```python
from build123d import *

# Parameters (mm, degrees)
SKETCH_1_W          = 56
SKETCH_1_H          = 85
SKETCH_1_R          = 1.5
EXTRUDE_1_DEPTH     = 1.28
FILLET_1_R          = 3
SKETCH_6_W          = 5
SKETCH_6_H          = 6
CUT_EXTRUDE_1_DEPTH = 2.28
SKETCH_4_W          = 8
SKETCH_4_H          = 10
EXTRUDE_2_DEPTH     = 6
SKETCH_5_W          = 9
SKETCH_5_H          = 4
EXTRUDE_3_DEPTH     = 3
SKETCH_2_W          = 13
SKETCH_2_H          = 13
EXTRUDE_4_DEPTH     = 7
SKETCH_3_W          = 7
SKETCH_3_H          = 8
EXTRUDE_5_DEPTH     = 3
SKETCH_7_W          = 1.5
SKETCH_7_H          = 1.5
EXTRUDE_6_DEPTH     = 2
EXTRUDE_START       = 37.5
EXTRUDE_8_DEPTH     = 67


with BuildPart() as part:
    # 草圖1 → 填料-伸長1 (new body)
    with BuildSketch(Plane(origin=(0, 0, 0), x_dir=(1, 0, 0), z_dir=(0, 1, 0))):
        Rectangle(SKETCH_1_W, SKETCH_1_H)
        with Locations((-24.5, 19)):
            Circle(SKETCH_1_R, mode=Mode.SUBTRACT)
        with Locations((-24.5, -39)):
            Circle(SKETCH_1_R, mode=Mode.SUBTRACT)
        with Locations((24.5, -39)):
            Circle(SKETCH_1_R, mode=Mode.SUBTRACT)
        with Locations((24.5, 19)):
            Circle(SKETCH_1_R, mode=Mode.SUBTRACT)
    extrude(amount=EXTRUDE_1_DEPTH)

    # 圓角1
    fillet_1_edges = [part.edges().sort_by_distance(p)[0] for p in [
        (28, 0.64, 42.5),
        (-28, 0.64, 42.5),
        (-28, 0.64, -42.5),
        (28, 0.64, -42.5),
    ]]
    fillet(fillet_1_edges, radius=FILLET_1_R)

    # 草圖6 → 除料-伸長1 (cut, through all)
    with BuildSketch(Plane(origin=(0, 1.28, 0), x_dir=(1, 0, 0), z_dir=(0, 1, 0))):
        with Locations((-23.1, -29.5)):
            Rectangle(SKETCH_6_W, SKETCH_6_H)
    extrude(amount=-CUT_EXTRUDE_1_DEPTH, mode=Mode.SUBTRACT)

    # 草圖4 → 填料-伸長2 (add)
    with BuildSketch(Plane(origin=(0, 1.28, 0), x_dir=(1, 0, 0), z_dir=(0, 1, 0))):
        with Locations((-16, 5)):
            Rectangle(SKETCH_4_W, SKETCH_4_H)
    extrude(amount=EXTRUDE_2_DEPTH)

    # 草圖5 → 填料-伸長3 (add)
    with BuildSketch(Plane(origin=(0, 1.28, 0), x_dir=(1, 0, 0), z_dir=(0, 1, 0))):
        with Locations((0, -37.5)):
            Rectangle(SKETCH_5_W, SKETCH_5_H)
    extrude(amount=EXTRUDE_3_DEPTH)

    # 草圖2 → 填料-伸長4 (add)
    with BuildSketch(Plane(origin=(0, 1.28, 0), x_dir=(1, 0, 0), z_dir=(0, 1, 0))):
        with Locations((21.5, -12)):
            Rectangle(SKETCH_2_W, SKETCH_2_H)
        with Locations((21.5, -29)):
            Rectangle(SKETCH_2_W, SKETCH_2_H)
    extrude(amount=EXTRUDE_4_DEPTH)

    # 草圖3 → 填料-伸長5 (add)
    with BuildSketch(Plane(origin=(0, 1.28, 0), x_dir=(1, 0, 0), z_dir=(0, 1, 0))):
        with Locations((24.5, 7.5)):
            Rectangle(SKETCH_3_W, SKETCH_3_H)
    extrude(amount=EXTRUDE_5_DEPTH)

    # 草圖7 → 填料-伸長6 (add)
    with BuildSketch(Plane.XY.offset(39.5)):
        with Locations((1.65, 3.13)):
            Rectangle(SKETCH_7_W, SKETCH_7_H)
    extrude(amount=EXTRUDE_6_DEPTH)

    # 草圖9 → 填料-伸長8 (add)
    with BuildSketch(Plane.XY.offset(EXTRUDE_START)):
        with BuildLine():
            Line((-16, 0), (16, 0))
            ThreePointArc((16, 0), (20.5, -4.5), (16, -9))
            Line((16, -9), (-16, -9))
            ThreePointArc((-16, -9), (-20.5, -4.5), (-16, 0))
        make_face()
    extrude(amount=-EXTRUDE_8_DEPTH)


solid = part.part
```
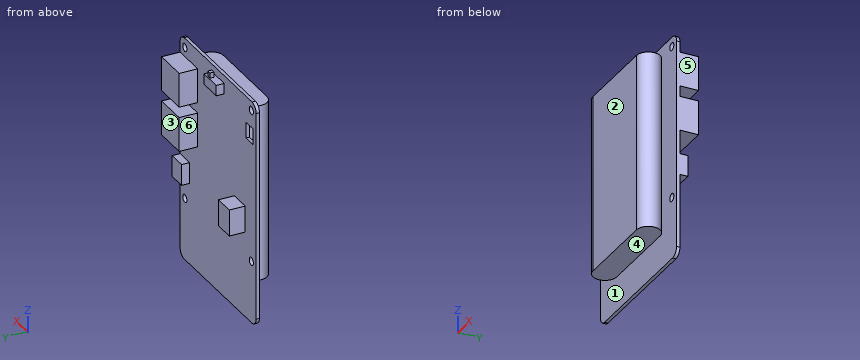
The listing builds one solid part. Answer for the finished solid, in the listing's coordinates (mm). Face numbers are marked on the shaded views. A direction names the side the tool comes from. Coordinates: 2 decimals unless noted, no trailing zeros. Write each loop counter-clockwise with the first axis right and the second up, starting at its lowest first coordinate (ties: lowest second). Pieces come first, ordered by that corner, then holes. Notation, with made-up numbers: (-40, 85.25) - (-14, 85.25) arc R31 cw to (-14, 118.25) - close; hole circle Ø10 at (-10, 20). An arc over 180 degrees is marked (long way). Return JSON: item names as keys, results as strings. Group by question number.
Q1. The part is cut by section D-D on x = 9.5. Write down the section's boundary in (y, z).
Q2. For a pull along Y with two mould halves and no side action, classify the marked faces 1, 2 and 3 as +Y half, -Y half, draft (parallel to the pull), parting line (faces both ways), or undercut.
Q3. Find the intervals of material crossed by line 1 along Z through (x, y) = (24.5, 0.4); line 2 along Z through (x, y) = (-24.5, 0.4); line 3 along X through (y, z) = (0.85, 39), in increasing order. Write a range as [from, to].
Q4. The part is cut by section B-B on x = -17. Write down the section's boundary in (y, z).
Q5. The part is cut by section A-A on z = 29. Write down the section's boundary in (x, y).
Q6. Flat-ended cylindrical pins translate along their axes: pin 1 Ø4.5 at (x, y) = (-8.5, -6.5) entering from -Z; pin 2 Ø4.5 at (x, y) = (6, -2.5) entering from +Z; pin 3 Ø1.5 at (x, y) = (0, 3.5) entering from +Z. Find the tip coordinate at first contact, or state that the pin passes through.
Q7. Which of the six approach directions +Z, -Z, +X, -X, +Y, -Y give full straight-line access (tool end or side, diameter ignored) to the marked faces 4, 5 and 6?
Q8. The part is cut by section C-C on z = 15.5. Write down the section's boundary in (x, y), and give its area (3 significant figures).
Evaluation:
{
 "1": {"outline": "(-9, -29.5) - (0, -29.5) - (0, -42.5) - (1.28, -42.5) - (1.28, 42.5) - (0, 42.5) - (0, 37.5) - (-9, 37.5) - close"},
 "2": {"face 1": "undercut", "face 2": "-Y half", "face 3": "+Y half"},
 "3": {"line 1": "z = [-42.5, -20.5], [-17.5, 37.5], [40.5, 42.5]", "line 2": "z = [-42.5, -20.5], [-17.5, 26.5], [32.5, 37.5], [40.5, 42.5]", "line 3": "x = [-28, -26], [-23, 23], [26, 28]"},
 "4": {"outline": "(-8.89, -29.5) - (-0.11, -29.5) - (-0.11, 37.5) - (-8.89, 37.5) - close; (0, -42.5) - (1.28, -42.5) - (1.28, -10) - (7.28, -10) - (7.28, 0) - (1.28, 0) - (1.28, 42.5) - (0, 42.5) - close"},
 "5": {"outline": "(-28, 0) - (-25.6, 0) - (-25.6, 1.28) - (-28, 1.28) - close; (-20.6, 0) - (-16, 0) arc R4.5 ccw to (-16, -9) - (16, -9) arc R4.5 ccw to (16, 0) - (28, 0) - (28, 8.28) - (15, 8.28) - (15, 1.28) - (-20.6, 1.28) - close"},
 "6": {"pin 1": "stops at z = -29.5", "pin 2": "stops at z = 37.5", "pin 3": "stops at z = 39.5"},
 "7": {"face 4": "-Z, +X, -X, -Y", "face 5": "+Z, -Z, +X, +Y, -Y", "face 6": "+Z, -Z, -X, +Y"},
 "8": {"outline": "(-28, 0) - (-16, 0) arc R4.5 ccw to (-16, -9) - (16, -9) arc R4.5 ccw to (16, 0) - (28, 0) - (28, 8.28) - (15, 8.28) - (15, 1.28) - (-28, 1.28) - close", "area": "514 mm2"}
}
